Geometry: final body of the model. Coordinates: model frame, mm. A direction names the side the tool comes from. Give positions to 0.01 mm unless a question says otherwise; leave off trailing zeros. Order: outer loops, then holes, each group sorted by start corner. A loop starts at its lowest first (then second) coordinate and runs counter-clockwise, first axis right, second up. Notation, with made-up numbers: M 57.25,74 L 91.25,74 A15 ccw 91.25,99 Z; hole C -10,80 d3. An arc over 180 degrees is marked long. Use CSV: the item, a comma, the result in double quotes.
```python
from build123d import *

# Parameters (mm, degrees)
F0_W     = 110
F0_H     = 10
F1_DEPTH = 3
F0_H_2   = 3
F3_DEPTH = 20
F2_W     = 20
F2_H     = 10
F4_DEPTH = 3
F6_DEPTH = 3


with BuildPart() as f1:
    # F0 (on Top) → F1 (new body)
    with BuildSketch(Plane.XY):
        Rectangle(F0_W, F0_H)
    extrude(amount=F1_DEPTH)

    # F0 (on Top) → F3 (join)
    with BuildSketch(Plane.XY):
        with Locations((0, -6.5)):
            Rectangle(F0_W, F0_H_2)
        with Locations((0, 6.5)):
            Rectangle(F0_W, F0_H_2)
    extrude(amount=F3_DEPTH)

    # F2 (on face) → F4 (cut, through all)
    with BuildSketch(Plane.XY.offset(3)):
        with Locations((-45, 0)):
            Rectangle(F2_W, F2_H)
    extrude(amount=-F4_DEPTH, mode=Mode.SUBTRACT)

    # F5 (on face) → F6 (join, through all)
    with BuildSketch(Plane.XY.offset(3)):
        with BuildLine():
            Line((-9.536225, -5), (-26.390179, -5))
            Line((-26.390179, -5), (-21.141226, -25.801912))
            ThreePointArc((-21.141226, -25.801912), (-17.963202, -28.277636), (-14.785178, -25.801912))
            Line((-14.785178, -25.801912), (-9.536225, -5))
        make_face()
        with BuildLine():
            Line((46.390179, -5), (29.536225, -5))
            Line((29.536225, -5), (34.785178, -25.801912))
            ThreePointArc((34.785178, -25.801912), (37.963202, -28.277636), (41.141226, -25.801912))
            Line((41.141226, -25.801912), (46.390179, -5))
        make_face()
        with BuildLine():
            Line((-21.141226, 25.801912), (-26.390179, 5))
            Line((-26.390179, 5), (-9.536225, 5))
            Line((-9.536225, 5), (-14.785178, 25.801912))
            ThreePointArc((-14.785178, 25.801912), (-17.963202, 28.277636), (-21.141226, 25.801912))
        make_face()
        with BuildLine():
            Line((34.785178, 25.801912), (29.536225, 5))
            Line((29.536225, 5), (46.390179, 5))
            Line((46.390179, 5), (41.141226, 25.801912))
            ThreePointArc((41.141226, 25.801912), (37.963202, 28.277636), (34.785178, 25.801912))
        make_face()
    extrude(amount=-F6_DEPTH)


solid = f1.part
```
1. Pull-direction query (X, two-part tool) for faces 6 (the face through (-23.356, 17.026, 1.521)), 7 (the face through (43.419, 16.776, 1.521)), 8 (the face through (-17.902, 28.277, 1.521)), 9 (the face through (32.51, -16.78, 1.52)); classes: +X half, -X half, draft (parallel to the pull), parting line (faces both ways), or undercut.
Answer:
face 6,"-X half"
face 7,"+X half"
face 8,"undercut"
face 9,"undercut"
2. Reachability of faces 1 (the face through (-12.51, 16.78, 1.52)), 2 (the face through (9, 0, 3)), 3 (the face through (-18, -16, 3)), 4 (the face through (-18, 16, 3)), 5 (the face through (-12.57, -17.03, 1.52)) from +Z, -Z, +X, -X, +Y, -Y: full face, straight path, thin tool, end or side. Return the list, or none.
Answer:
face 1,"+Z, -Z, +Y"
face 2,"+Z, +X, -X"
face 3,"+Z, +X, -X, -Y"
face 4,"+Z, +X, -X, +Y"
face 5,"+Z, -Z, -Y"
3. Pin query (flat end, axial travel): pin 1 Ø10 at (x, z) = (-11, 9.5) entering from -Y; pin 2 Ø1.5 at (y, z) = (2.5, 1) entering from -X; pin 3 Ø12 at (x, z) = (6.5, 7) entering from +Y. Return the tip coordinate at first contact, or that it passes through.
Answer:
pin 1,"y = -8"
pin 2,"x = -35"
pin 3,"y = 8"
4. Section A-A, the plane z = 16.25. Return the cut outline in (x, y), plus the area to 3 significant figures.
Answer:
outline,"M -55,-8 L 55,-8 L 55,-5 L -55,-5 Z; M -55,5 L 55,5 L 55,8 L -55,8 Z"
area,"660 mm2"
5. Line query: line 1 (Y direction, x = 30, z = 8); line 2 (Z direction, x = 43, y = 0); line 3 (Y direction, x = 48, z = 1). Output: solid intervals per line, ascending.
Answer:
line 1,"-8 to -5, 5 to 8"
line 2,"0 to 3"
line 3,"-8 to 8"
6. Section C-C, the plane x = -2. Return the cut outline in (y, z).
Answer:
outline,"M -8,0 L 8,0 L 8,20 L 5,20 L 5,3 L -5,3 L -5,20 L -8,20 Z"
7. Section D-D, the plane y = -2. Return the cut outline in (x, z), plus the area to 3 significant figures.
Answer:
outline,"M -35,0 L 55,0 L 55,3 L -35,3 Z"
area,"270 mm2"
8. Section B-B, the plane y = -16. Return the cut outline in (x, z), plus the area to 3 significant figures.
Answer:
outline,"M -23.61,0 L -12.31,0 L -12.31,3 L -23.61,3 Z; M 32.31,0 L 43.61,0 L 43.61,3 L 32.31,3 Z"
area,"67.8 mm2"
